```python
from build123d import *

# Parameters (mm, degrees)
BOSS_EXTRUDE1_DEPTH      = 2
BOSS_EXTRUDE1_DEPTH_BACK = 2
SKETCH2_R                = 1.7
FILLET1_R                = 20
SKETCH7_R                = 6
SKETCH7_R_2              = 1.7
BOSS_EXTRUDE4_DEPTH      = 4
SKETCH8_R                = 3.7
SKETCH8_R_2              = 1.7
BOSS_EXTRUDE5_DEPTH      = 2
FILLET4_R                = 2


with BuildPart() as part:
    # Sketch2 → Boss-Extrude1 (new, two sides: drawn at the far end of the back side and taken through both)
    with BuildSketch(Plane.XY.offset(-BOSS_EXTRUDE1_DEPTH_BACK)):
        with BuildLine():
            Line((1.575752274, -4.745208612), (34.456924853, 5.232629629))
            Line((34.456924853, 5.232629629), (44.296635241, 16.864742156))
            ThreePointArc((44.296635241, 16.864742156), (46.218376178, 23.740514028), (40.203783054, 27.586810508))
            Line((40.203783054, 27.586810508), (7.512886707, 26.600773906))
            ThreePointArc((7.512886707, 26.600773906), (2.79322071, 19.950091357), (10.629154827, 17.690675057))
            Line((10.629154827, 17.690675057), (25.733767379, 18.146266751))
            Line((25.733767379, 18.146266751), (18.728666276, 9.86511608))
            Line((18.728666276, 9.86511608), (1.70658462, 4.699741369))
            ThreePointArc((1.70658462, 4.699741369), (-4.999520368, 0.069253832), (1.575752274, -4.745208612))
        make_face()
        Circle(SKETCH2_R, mode=Mode.SUBTRACT)
        with Locations((40.612886707, 21.600773906)):
            Circle(SKETCH2_R, mode=Mode.SUBTRACT)
        with Locations((7.512886707, 21.600773906)):
            Circle(SKETCH2_R, mode=Mode.SUBTRACT)
    extrude(amount=BOSS_EXTRUDE1_DEPTH + BOSS_EXTRUDE1_DEPTH_BACK)

    # Fillet1
    fillet1_edges = [part.edges().sort_by_distance(p)[0] for p in [
        (34.456924853, 5.232629629, 0),
        (18.728666276, 9.86511608, 0),
    ]]
    fillet(fillet1_edges, radius=FILLET1_R)

    # Sketch7 → Boss-Extrude4 (add)
    with BuildSketch(Plane(origin=(0, 0, 2), x_dir=(-1, 0, 0), z_dir=(0, 0, -1))):
        with Locations(Location((-40.612886707, 21.600773906, 0), (0, 0, 232.123747861))):
            Circle(SKETCH7_R)
        with Locations(Location((-40.612886707, 21.600773906, 0), (0, 0, 180))):
            Circle(SKETCH7_R_2, mode=Mode.SUBTRACT)
    extrude(amount=-BOSS_EXTRUDE4_DEPTH)

    # Sketch8 → Boss-Extrude5 (add)
    # profile 1 of 2: a face of its own
    with BuildSketch(Plane(origin=(0, 0, 2), x_dir=(-1, 0, 0), z_dir=(0, 0, -1))):
        with Locations((-7.512886707, 21.600773906)):
            Circle(SKETCH8_R)
        with Locations(Location((-7.512886707, 21.600773906, 0), (0, 0, 180))):
            Circle(SKETCH8_R_2, mode=Mode.SUBTRACT)
    # profile 2 of 2: a face of its own
    with BuildSketch(Plane(origin=(0, 0, 2), x_dir=(-1, 0, 0), z_dir=(0, 0, -1))):
        Circle(SKETCH8_R)
        with Locations(Location((0, 0, 0), (0, 0, 180))):
            Circle(SKETCH8_R_2, mode=Mode.SUBTRACT)
    extrude(amount=-BOSS_EXTRUDE5_DEPTH)

    # Fillet4
    fillet4_edges = [part.edges().sort_by_distance(p)[0] for p in [
        (25.733767379, 18.146266751, 0),
    ]]
    fillet(fillet4_edges, radius=FILLET4_R)


solid = part.part
```
Can you work these out from the model? Positions are in its coordinate system, mm. A direction names the side the tool comes from. Round coordinates to 2 decimals unless told otherwise and drop trailing zeros. Order: outer loops, then holes, each group sorted by start corner. A loop starts at its lowest first (then second) coordinate and runs counter-clockwise, first axis right, second up.
(1) If we section it at D-D (y = 0): Please give me the cut outline in (x, z), plus the area to 3 significant figures.
Results are:
outline: (-5, -2) - (-1.7, -2) - (-1.7, 4) - (-3.7, 4) - (-3.7, 2) - (-5, 2) - close; (1.7, -2) - (17.21, -2) - (17.21, 2) - (3.7, 2) - (3.7, 4) - (1.7, 4) - close
area: 83.3 mm2
(2) If we section it at C-C (x = 6.5): Please give me the cut outline in (y, z), plus the area to 3 significant figures.
Results are:
outline: (-3.25, -2) - (6.15, -2) - (6.15, 2) - (-3.25, 2) - close; (16.7, -2) - (20.24, -2) - (20.24, 4) - (18.04, 4) - (18.04, 2) - (16.7, 2) - close; (22.97, -2) - (26.5, -2) - (26.5, 2) - (25.16, 2) - (25.16, 4) - (22.97, 4) - close
area: 74.6 mm2
(3) If I drill on L1, parallel to Y at x = 8, z = 1.75; L2, parallel to X at y = 23, z = -1; L3, parallel to Z at x = 16, y = 9, over which ranges is the centre line in solid material (lowest first)?
Results are:
L1: y = -2.8 to 6.61, 16.62 to 19.97, 23.23 to 26.62
L2: x = 2.71 to 6.55, 8.48 to 39.65, 41.58 to 46.45
L3: z = -2 to 2
(4) If we section it at A-A (x = 0): Please give me the cut outline in (y, z), plus the area to 3 significant figures.
Results are:
outline: (-5, -2) - (-1.7, -2) - (-1.7, 4) - (-3.7, 4) - (-3.7, 2) - (-5, 2) - close; (1.7, -2) - (5, -2) - (5, 2) - (3.7, 2) - (3.7, 4) - (1.7, 4) - close
area: 34.4 mm2
(5) We'd pull the mould along X, two halves only. Please class faces 1 (the face through (41.24, 13.25, -0.03)), 2 (the face through (23.1, 16.9, 0)), 3 (the face through (-1, -2, 4)): +X half, -X half, draft (parallel to the pull), parting line (faces both ways), or undercut.
Results are:
face 1: +X half
face 2: undercut
face 3: draft
(6) I'm going to push flat-ended pins straight in: pin 1 (5 mm diameter, centred on x = 29, y = 22, fed in from +Z); pin 2 (4.5 mm diameter, centred on x = 40.61, y = 21.6, fed in from +Z); pin 3 (1 mm diameter, centred on y = 7.5, z = 4, fed in from +X); pin 4 (3.5 mm diameter, centred on x = -0.5, y = -1.5, fed in from +Z). Where does each tip first touch, or does it pass through?
Results are:
pin 1: stops at z = 2
pin 2: stops at z = 6
pin 3: passes through
pin 4: stops at z = 4
(7) If we section it at B-B (z = 3): Please give me the cut outline in (x, y).
Results are:
outline: circle Ø7.4 at (0, 0); circle Ø7.4 at (7.51, 21.6); circle Ø12 at (40.61, 21.6); hole circle Ø3.4 at (0, 0); hole circle Ø3.4 at (7.51, 21.6); hole circle Ø3.4 at (40.61, 21.6)
(8) On a 3-axis mill with a long thin cutter (end or side, diameter ignored), from which of +Z, -Z, +X, -X, +Y, -Y can I reach the whole of each face in a straight line? I mean faces 4 (the face through (9.2, 20.8, 4)), 5 (the face through (18.19, 10.53, 0.03)), 6 (the face through (42.183, 22.252, 1.944)), 7 (the face through (10.24, 24.1, 2.99)). Say none if no direction works.
Results are:
face 4: +Z, -X, +Y, -Y
face 5: +Z, -Z, -X
face 6: +Z, -Z
face 7: +Z
